from build123d import *

# Parameters (mm, degrees)
F0_R     = 7.5
F0_R_2   = 5.25
F1_DEPTH = 14
F2_R     = 1
F3_R     = 0.5


with BuildPart() as f1:
    # F0 (on Right) → F1 (new body)
    with BuildSketch(Plane.YZ):
        Circle(F0_R)
        Circle(F0_R_2, mode=Mode.SUBTRACT)
    extrude(amount=F1_DEPTH)

    # F2
    f2_edges = [f1.edges().sort_by_distance(p)[0] for p in [
        (0, -7.5, 0),
        (14, -7.5, 0),
    ]]
    fillet(f2_edges, radius=F2_R)

    # F3
    f3_edges = [f1.edges().sort_by_distance(p)[0] for p in [
        (14, -5.25, 0),
        (7, 5.25, 0),
        (0, -5.25, 0),
    ]]
    fillet(f3_edges, radius=F3_R)


solid = f1.part
Design review of the part built by this model. Coordinates are the model's own, in mm. Give positions to 0.01 mm unless a question says otherwise; leave off trailing zeros. Loops run counter-clockwise (first coordinate to the right, second up) from the corner with the lowest first, then second, coordinate; pieces in that order, holes last. Notation, with made-up numbers: (72, 63) - (84, 63) arc R7 cw to (84, 70) - close; hole circle Ø2 at (-37.5, 25). An arc over 180 degrees is marked (long way). Write item = value, one per line.
1) Clearance check with flat-ended pins moving along their axes: pin 1 Ø3 at (x, y) = (2, 1.5) entering from -Z; pin 2 Ø8.5 at (y, z) = (0, 0) entering from -X; pin 3 Ø3 at (x, z) = (7.5, -6) entering from +Y; pin 4 Ø1.5 at (x, y) = (4, -1.5) entering from +Z. State where each tip first meets the part, or that it passes through.
Result sheet:
pin_1 = -7.5
pin_2 = through
pin_3 = 6
pin_4 = 7.46
2) Take a section at A-A on z = 0. State the section outline as (x, y) points.
Result sheet:
outline = (0, -6.5) arc R1 ccw to (1, -7.5) - (13, -7.5) arc R1 ccw to (14, -6.5) - (14, -5.75) arc R0.5 ccw to (13.5, -5.25) - (0.5, -5.25) arc R0.5 ccw to (0, -5.75) - close; (0, 5.75) arc R0.5 ccw to (0.5, 5.25) - (13.5, 5.25) arc R0.5 ccw to (14, 5.75) - (14, 6.5) arc R1 ccw to (13, 7.5) - (1, 7.5) arc R1 ccw to (0, 6.5) - close
3) Draft analysis for pull direction Z (two halves, no side actions). For faces 1 (the face through (6.916, -7.493, 0.33)), 2 (the face through (0, 0, -6)), 3 (the face through (6.9, 5, 1.6)), state which applies: +Z half, -Z half, draft (parallel to the pull), parting line (faces both ways), or undercut.
Result sheet:
face_1 = parting line
face_2 = draft
face_3 = undercut
4) To check wall thickness, follow line 1 (Z direction, x = 5, y = 0); line 2 (Y direction, x = 6.25, z = -1.25); line 3 (Y direction, x = 4.25, z = 3). State the ranges of each line that lie inside material, in increasing order.
Result sheet:
line_1 = -7.5 to -5.25, 5.25 to 7.5
line_2 = -7.4 to -5.1, 5.1 to 7.4
line_3 = -6.87 to -4.31, 4.31 to 6.87
5) Take a section at C-C on x = 8.75. State the section outline as (y, z) points.
Result sheet:
outline = circle Ø15 at (0, 0); hole circle Ø10.5 at (0, 0)
